The listing builds one solid part. Answer for the finished solid, in the listing's coordinates (mm). Face numbers are marked on the shaded views. A direction names the side the tool comes from. Coordinates: 2 decimals unless noted, no trailing zeros.
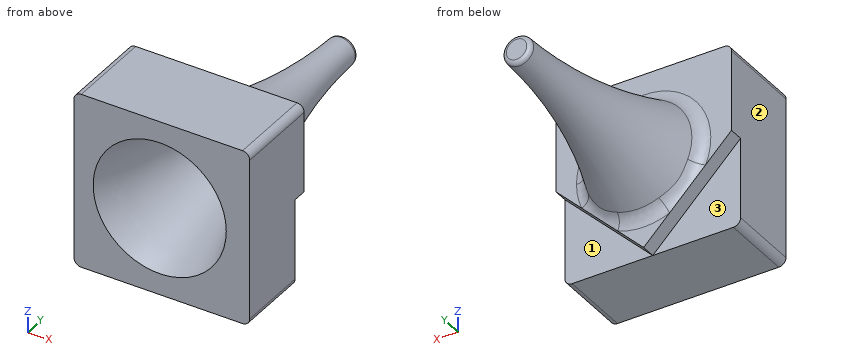
from build123d import *

# Parameters (mm, degrees)
ESQUISSE1_W             = 12.2
ESQUISSE1_H             = 12.2
BOSS_EXTRU_1_DEPTH      = 6
ENL_V_MAT_EXTRU_1_DEPTH = 1
CONG_2_R                = 0.3
CONG_3_R                = 0.5
CONG_4_R                = 1


with BuildPart() as part:
    # Esquisse1 → Boss.-Extru.1 (new body)
    with BuildSketch(Plane(origin=(0, 0, 0), x_dir=(1, 0, 0), z_dir=(0, 1, 0))):
        Rectangle(ESQUISSE1_W, ESQUISSE1_H)
    extrude(amount=BOSS_EXTRU_1_DEPTH)

    # Esquisse2 → Enlèv. mat.-Extru.1 (cut)
    with BuildSketch(Plane(origin=(0, 6, 0), x_dir=(1, 0, 0), z_dir=(0, 1, 0))):
        Polygon((-6.1, 6.1), (-6.1, 0), (0, 6.1), align=None)
        Polygon((6.1, 6.1), (0, 6.1), (6.1, 0), align=None)
    extrude(amount=-ENL_V_MAT_EXTRU_1_DEPTH, mode=Mode.SUBTRACT)

    # Esquisse4 → Révolution1 (revolve)
    with BuildSketch(Plane.XY):
        with BuildLine():
            Line((0, 20), (0, 6))
            Line((0, 6), (4, 6))
            add(Edge.make_bspline(
                [(4, 6), (1.118476113, 12.647093335), (1, 20)],
                knots=[0, 0, 0, 1, 1, 1], degree=2))
            Line((1, 20), (0, 20))
        make_face()
    revolve(axis=Axis((0, 20, 0), (0, -1, 0)))

    # Congé2
    cong_2_edges = [part.edges().sort_by_distance(p)[0] for p in [
        (-1, 20, 0),
    ]]
    fillet(cong_2_edges, radius=CONG_2_R)

    # Congé3
    cong_3_edges = [part.edges().sort_by_distance(p)[0] for p in [
        (-6.1, 2.5, -6.1),
        (6.1, 2.5, -6.1),
        (6.1, 3, 6.1),
        (-6.1, 3, 6.1),
    ]]
    fillet(cong_3_edges, radius=CONG_3_R)

    # Esquisse5 → Enlèvement de matière-Révolution1 (revolve, cut)
    with BuildSketch(Plane.XY):
        with BuildLine():
            Line((-0.15, 17), (-0.15, 0))
            Line((-0.15, 0), (4.472372581, 0))
            add(Edge.make_bspline(
                [(4.472372581, 0), (2.630008633, 3.831055764), (1.072108734, 14.115127784), (0.713133272, 17)],
                knots=[0, 0, 0, 0, 1, 1, 1, 1], degree=3))
            Line((0.713133272, 17), (-0.15, 17))
        make_face()
    revolve(axis=Axis((-0.15, 17, 0), (0, -1, 0)), mode=Mode.SUBTRACT)

    # Congé4
    cong_4_edges = [part.edges().sort_by_distance(p)[0] for p in [
        (-4, 6, 0),
    ]]
    fillet(cong_4_edges, radius=CONG_4_R)


solid = part.part
Q1. Which of the six approach directions +Z, -Z, +X, -X, +Y, -Y give full straight-line access (tool end or side, diameter ignored) to the marked faces 1, 2 and 3?
Answers below:
face 1: -Z, +X, +Y
face 2: +Z, -Z, -X, +Y, -Y
face 3: -Z, -X, +Y
Q2. Given pin 1 (1.8 mm diameter, centred on x = -2.5, z = -4.5, fed in from +Y); pin 2 (5 mm diameter, centred on x = -3, y = 9, fed in from -Z); pin 3 (1.4 mm diameter, centred on x = -1, z = -5.5, fed in from +Y); pin 4 (4 mm diameter, centred on x = -3.5, y = 15.5, fed in from -Z), each flat-ended and moving along its own axis, determine where each tip first touches the part or whether it passes through.
Answers below:
pin 1: stops at y = 6.08
pin 2: stops at z = -3.27
pin 3: stops at y = 6
pin 4: passes through
Q3. Find the intervals of material crossed by probe 1 along Y at (x, z) = (-5.5, 1.25); probe 2 along Y at (x, z) = (0, -0.25); probe 3 along X at (y, z) = (1, 1), in increasing order.
Answers below:
probe 1: y = 0 to 6
probe 2: y = 17 to 20
probe 3: x = -6.1 to -4.23, 3.93 to 6.1
